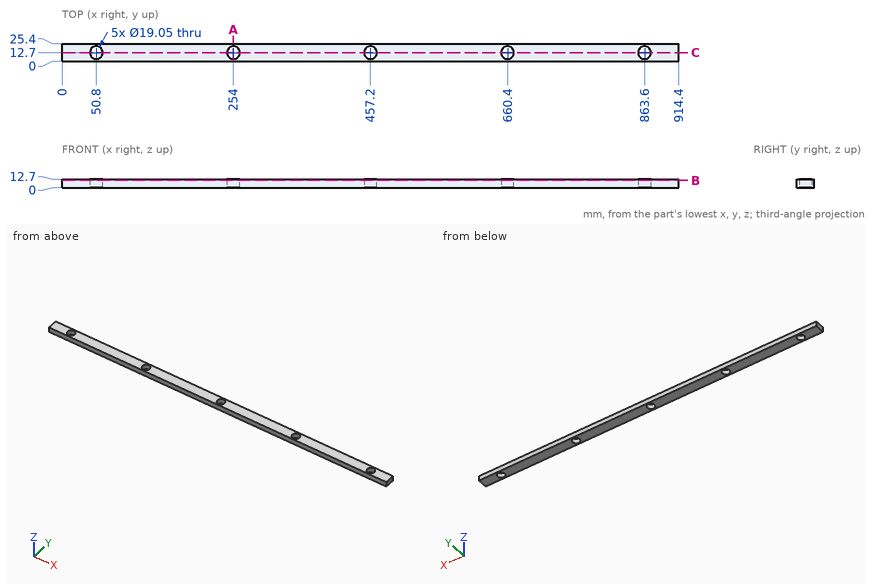
Study the drawing (mm; zero at the part's minimum x, y, z) and answer. Coordinates: 2 decimals unless noted, no trailing zeros. Loops run counter-clockwise (first coordinate to the right, second up) from the corner with the lowest first, then second, coordinate; pieces in that order, holes last. Notation, with made-up numbers: M 45.25,83 L 95.25,83 A14 cw 95.25,91 Z; hole C 2.5,4.25 d9. An arc over 180 degrees is marked long. Answer as a JSON object with one key per item and string values. Group by question number.
Item 1: Section A-A (x = 254) is taken. Write down the section's boundary in (y, z) (3 decimals), and give its area (3 significant figures).
Item 2: Consider L1, parallel to X at y = 13, z = 10.5; L2, parallel to Y at x = 863.6, z = 5 (3 decimals); L3, parallel to X at y = 14, z = 4.25. Determine where each line is inside the solid, lowest interval first.
Item 3: Section C-C (y = 12.7) is taken. Write down the section's boundary in (x, z) (3 decimals), and give its area (3 significant figures).
Item 4: Section B-B (z = 10.75) is taken. Write down the section's boundary in (x, y) (3 decimals), and give its area (3 significant figures).
Solved:
{
 "1": {"outline": "M 0,0 L 3.175,0 L 3.175,12.7 L 0,12.7 Z; M 22.225,0 L 25.4,0 L 25.4,12.7 L 22.225,12.7 Z", "area": "80.6 mm2"},
 "2": {"L1": "x = 0 to 41.28, 60.32 to 244.48, 263.52 to 447.68, 466.72 to 650.88, 669.92 to 854.08, 873.12 to 914.4", "L2": "y = 0 to 3.175, 22.225 to 25.4", "L3": "x = 0 to 41.36, 60.24 to 244.56, 263.44 to 447.76, 466.64 to 650.96, 669.84 to 854.16, 873.04 to 914.4"},
 "3": {"outline": "M 0,0 L 41.275,0 L 41.275,12.7 L 0,12.7 Z; M 60.325,0 L 244.475,0 L 244.475,12.7 L 60.325,12.7 Z; M 263.525,0 L 447.675,0 L 447.675,12.7 L 263.525,12.7 Z; M 466.725,0 L 650.875,0 L 650.875,12.7 L 466.725,12.7 Z; M 669.925,0 L 854.075,0 L 854.075,12.7 L 669.925,12.7 Z; M 873.125,0 L 914.4,0 L 914.4,12.7 L 873.125,12.7 Z", "area": "10,400 mm2"},
 "4": {"outline": "M 0,0 L 914.4,0 L 914.4,25.4 L 0,25.4 Z; hole C 50.8,12.7 d19.05; hole C 254,12.7 d19.05; hole C 457.2,12.7 d19.05; hole C 660.4,12.7 d19.05; hole C 863.6,12.7 d19.05", "area": "21,800 mm2"}
}
